The figure shows three views and two pictorial views of one solid part (mm, origin at its lowest corner). Answer the questions. Round coordinates to 2 decimals unless told otherwise and drop trailing zeros. Write each loop counter-clockwise with the first axis right and the second up, starting at its lowest first coordinate (ties: lowest second). Pieces come first, ordered by that corner, then holes. Notation, with made-up numbers: M 38.5,39 L 82.5,39 A11 cw 82.5,56 Z; hole C 5.5,83 d4. An arc over 180 degrees is marked long. Answer in a Markdown table with one row per item.
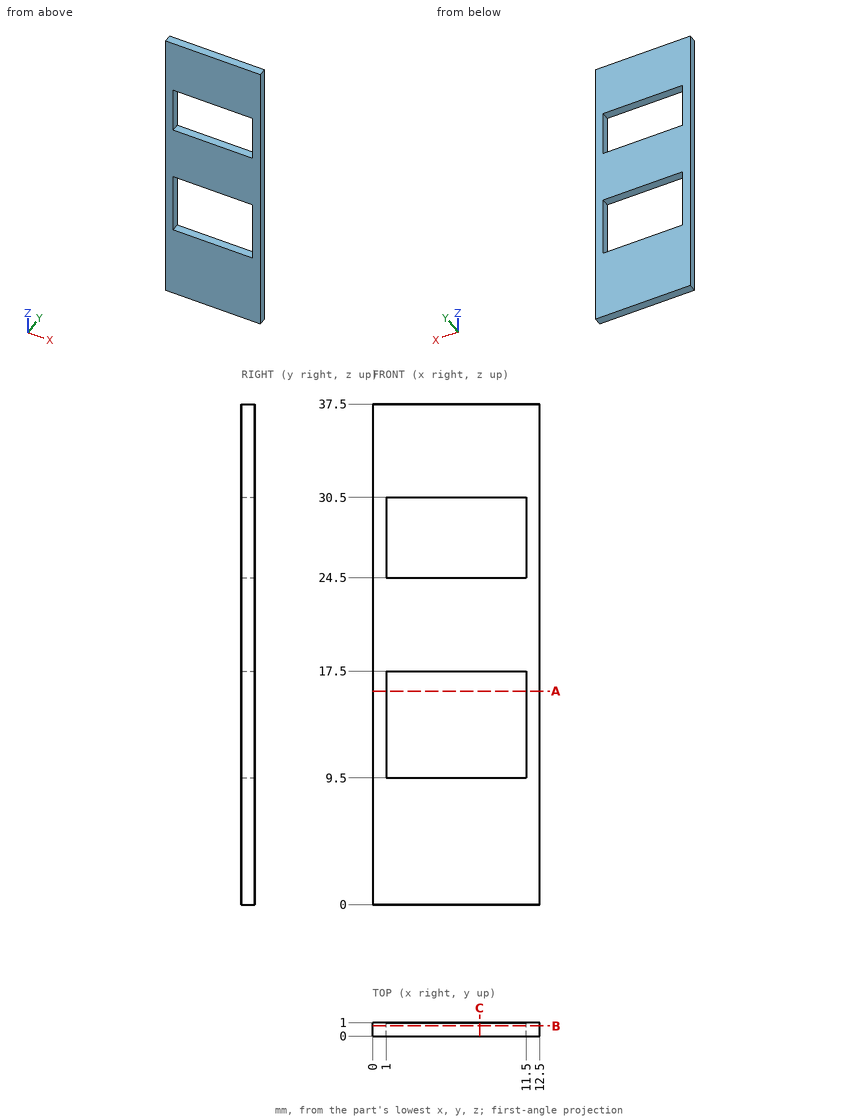
1. The part is cut by section A-A (z = 16). Determine the outline of the cut face in (x, y).
Calculated:
| item | result |
|---|---|
| outline | M 0,0 L 1,0 L 1,1 L 0,1 Z; M 11.5,0 L 12.5,0 L 12.5,1 L 11.5,1 Z |
2. The part is cut by section C-C (x = 8). Determine the outline of the cut face in (y, z), plus the area to 3 significant figures.
Calculated:
| item | result |
|---|---|
| outline | M 0,0 L 1,0 L 1,9.5 L 0,9.5 Z; M 0,17.5 L 1,17.5 L 1,24.5 L 0,24.5 Z; M 0,30.5 L 1,30.5 L 1,37.5 L 0,37.5 Z |
| area | 23.5 mm² |
3. Given pin 1 (2 mm diameter, centred on x = 10, z = 30, fed in from +Y), flat-ended and moving along its own axis, determine where the tip first touches the part or whether it passes through.
Calculated:
| item | result |
|---|---|
| pin 1 | stops at y = 1 |
4. The part is cut by section B-B (y = 0.75). Determine the outline of the cut face in (x, z).
Calculated:
| item | result |
|---|---|
| outline | M 0,0 L 12.5,0 L 12.5,37.5 L 0,37.5 Z; hole M 1,9.5 L 11.5,9.5 L 11.5,17.5 L 1,17.5 Z; hole M 1,24.5 L 11.5,24.5 L 11.5,30.5 L 1,30.5 Z |
5. Consider line 1 along Z through (x, y) = (1.5, 0.35); line 2 along X through (y, z) = (0.1, 26). Determine where each line is inside the solid, lowest interval first. Write a range as from..to.
Calculated:
| item | result |
|---|---|
| line 1 | z = 0..9.5, 17.5..24.5, 30.5..37.5 |
| line 2 | x = 0..1, 11.5..12.5 |
